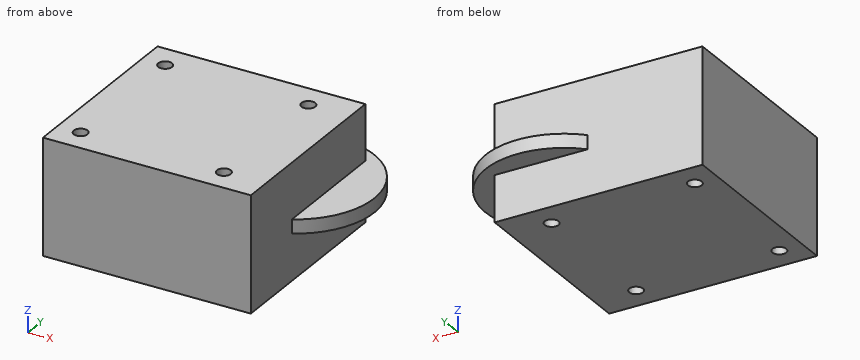
```python
from build123d import *

# Parameters (mm, degrees)
SKETCH1_W           = 45
SKETCH1_H           = 42
BOSS_EXTRUDE1_DEPTH = 25
SKETCH2_R           = 1.5
CUT_EXTRUDE1_DEPTH  = 26
SKETCH3_R           = 17
BOSS_EXTRUDE2_DEPTH = 3


with BuildPart() as part:
    # Sketch1 → Boss-Extrude1 (new body)
    with BuildSketch(Plane.XY):
        Rectangle(SKETCH1_W, SKETCH1_H)
    extrude(amount=BOSS_EXTRUDE1_DEPTH)

    # Sketch2 → Cut-Extrude1 (cut, through all)
    with BuildSketch(Plane.XY.offset(25)):
        with Locations((13.5, 15.35)):
            Circle(SKETCH2_R)
        with Locations((-17.5, 15.35)):
            Circle(SKETCH2_R)
        with Locations((-17.5, -15.65)):
            Circle(SKETCH2_R)
        with Locations((13.5, -15.65)):
            Circle(SKETCH2_R)
    extrude(amount=-CUT_EXTRUDE1_DEPTH, mode=Mode.SUBTRACT)

    # Sketch3 → Boss-Extrude2 (add)
    with BuildSketch(Plane.XY.offset(10)):
        with Locations((14.5, 9.06439174)):
            Circle(SKETCH3_R)
    extrude(amount=BOSS_EXTRUDE2_DEPTH)


solid = part.part
```
Read the model definition and answer for the solid it produces. Units are mm, in the model's axes. Give positions to 0.01 mm unless a question says otherwise; leave off trailing zeros. Order: outer loops, then holes, each group sorted by start corner. A loop starts at its lowest first (then second) coordinate and runs counter-clockwise, first axis right, second up.
(1) Given pin 1 (0.9 mm diameter, centred on x = 14, y = 16, fed in from +Z); pin 2 (1 mm diameter, centred on x = 13, y = 2.5, fed in from -Z); pin 3 (8 mm diameter, centred on x = 19, z = 3, fed in from +Y); pin 4 (8 mm diameter, centred on y = 4, z = 20.5, fed in from +X), each flat-ended and moving along its own axis, determine where each tip first touches the part or whether it passes through.
(2) Find section C-C (z = 16.25). Give the vertices of the cut face in (x, y), plus the area to 3 significant figures.
(3) Find section B-B (y = -15.65). Give the vertices of the cut face in (x, z).
(4) Find section D-D (y = 15.35). Give the vertices of the cut face in (x, z), plus the area to 3 significant figures.
(5) Find section A-A (x = -17.5). Give the vertices of the cut face in (y, z).
(6) Straight lines are drawn through the part: L1, parallel to Y at x = 13.5, z = 6; L2, parallel to X at y = 10, z = 5; L3, parallel to Y at x = 0, z = 7.25. For each, find the intervals that lie inside material, in ascending order.
Result sheet:
1. pin 1: stops at z = 13
1. pin 2: stops at z = 0
1. pin 3: stops at y = 21
1. pin 4: stops at x = 22.5
2. outline: (-22.5, -21) - (22.5, -21) - (22.5, 21) - (-22.5, 21) - close; hole circle Ø3 at (-17.5, -15.65); hole circle Ø3 at (-17.5, 15.35); hole circle Ø3 at (13.5, -15.65); hole circle Ø3 at (13.5, 15.35)
2. area: 1,860 mm2
3. outline: (-22.5, 0) - (-19, 0) - (-19, 25) - (-22.5, 25) - close; (-16, 0) - (12, 0) - (12, 25) - (-16, 25) - close; (15, 0) - (22.5, 0) - (22.5, 25) - (15, 25) - close
4. outline: (-22.5, 0) - (-19, 0) - (-19, 25) - (-22.5, 25) - close; (-16, 0) - (12, 0) - (12, 10) - (15, 10) - (15, 0) - (22.5, 0) - (22.5, 10) - (30.3, 10) - (30.3, 13) - (22.5, 13) - (22.5, 25) - (15, 25) - (15, 13) - (12, 13) - (12, 25) - (-16, 25) - close
4. area: 1,010 mm2
5. outline: (-21, 0) - (-17.15, 0) - (-17.15, 25) - (-21, 25) - close; (-14.15, 0) - (13.85, 0) - (13.85, 25) - (-14.15, 25) - close; (16.85, 0) - (21, 0) - (21, 25) - (16.85, 25) - close
6. L1: y = -21 to -17.15, -14.15 to 13.85, 16.85 to 21
6. L2: x = -22.5 to 22.5
6. L3: y = -21 to 21
